```python
from build123d import *

# Parameters (mm, degrees)
F0_W     = 482.6
F0_H     = 88.9
F1_DEPTH = 3
F2_R     = 3
F3_R     = 2.38125
F3_R_2   = 2.246181
F3_R_3   = 2.383077
F3_R_4   = 4.622163
F3_R_5   = 4.540173
F3_R_6   = 3.175
F3_R_7   = 4.7625
F4_DEPTH = 3


with BuildPart() as f1:
    # F0 (on Front) → F1 (new body)
    with BuildSketch(Plane.XZ):
        with Locations((0.070956, -0.013071)):
            Rectangle(F0_W, F0_H)
    extrude(amount=-F1_DEPTH)

    # F2
    f2_edges = [f1.edges().sort_by_distance(p)[0] for p in [
        (-241.229044, 1.5, 44.436929),
        (241.370956, 1.5, 44.436929),
        (241.370956, 1.5, -44.463071),
        (-241.229044, 1.5, -44.463071),
    ]]
    fillet(f2_edges, radius=F2_R)

    # F3 (on Front) → F4 (cut, through all)
    with BuildSketch(Plane.XZ):
        with BuildLine():
            Line((-234.3, 19.186929), (-230.8, 19.186929))
            ThreePointArc((-230.8, 19.186929), (-227.4, 22.586929), (-230.8, 25.986929))
            Line((-230.8, 25.986929), (-234.3, 25.986929))
            ThreePointArc((-234.3, 25.986929), (-237.7, 22.586929), (-234.3, 19.186929))
        make_face()
        with BuildLine():
            ThreePointArc((230.8, 25.986929), (227.4, 22.586929), (230.8, 19.186929))
            Line((230.8, 19.186929), (234.3, 19.186929))
            ThreePointArc((234.3, 19.186929), (237.7, 22.586929), (234.3, 25.986929))
            Line((234.3, 25.986929), (230.8, 25.986929))
        make_face()
        with BuildLine():
            Line((230.8, -25.986929), (234.3, -25.986929))
            ThreePointArc((234.3, -25.986929), (237.7, -22.586929), (234.3, -19.186929))
            Line((234.3, -19.186929), (230.8, -19.186929))
            ThreePointArc((230.8, -19.186929), (227.4, -22.586929), (230.8, -25.986929))
        make_face()
        with BuildLine():
            ThreePointArc((-230.8, -25.986929), (-227.4, -22.586929), (-230.8, -19.186929))
            Line((-230.8, -19.186929), (-234.3, -19.186929))
            ThreePointArc((-234.3, -19.186929), (-237.7, -22.586929), (-234.3, -25.986929))
            Line((-234.3, -25.986929), (-230.8, -25.986929))
        make_face()
        with Locations((-133.35, 13.767754)):
            Circle(F3_R)
        with Locations((-133.35, -5.282246)):
            Circle(F3_R_2)
        with Locations((-133.35, -17.982246)):
            Circle(F3_R_3)
        with Locations((-101.6, -11.684)):
            Circle(F3_R_4)
        with Locations((-82.55, -11.684)):
            Circle(F3_R_5)
        with Locations((-44.45, -11.684)):
            Circle(F3_R_6)
        with Locations((-6.35, -11.684)):
            Circle(F3_R_7)
        with Locations((25.4, -11.684)):
            Circle(F3_R_6)
        with Locations((50.8, -11.684)):
            Circle(F3_R_6)
        with Locations((76.2, -11.684)):
            Circle(F3_R_6)
        with Locations((107.95, -11.684)):
            Circle(F3_R_7)
        with Locations((146.05, -11.684)):
            Circle(F3_R_7)
    extrude(amount=-F4_DEPTH, mode=Mode.SUBTRACT)


solid = f1.part
```
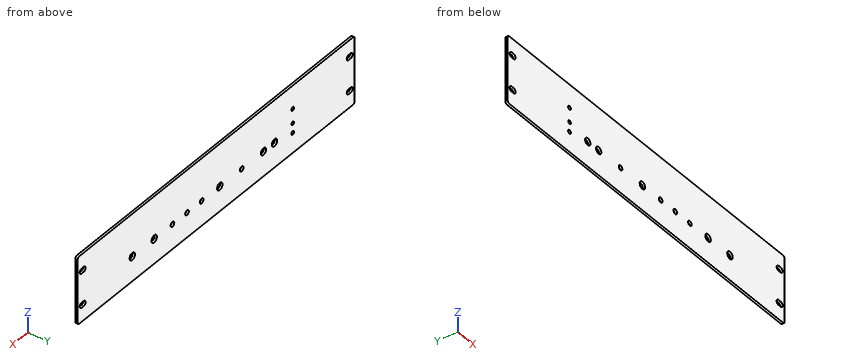
Check sheet for the modelled part. Datum: model origin and axes. Units: mm. Coordinates: 2 decimals unless noted, no trailing zeros. Write each loop counter-clockwise with the first axis right and the second up, starting at its lowest first coordinate (ties: lowest second). Pieces come first, ordered by that corner, then holes. Notation, with made-up numbers: M -22.5,52.25 L 33.5,52.25 A27 cw 33.5,76.25 Z; hole C 39,3 d7. An arc over 180 degrees is marked long. Write item = value, one per line. Start each with the question number.
1. Go/stop test with a flat-tipped pin: pin 1 (3 mm diameter, centred on x = -133.35, z = 13.77, fed in from +Y) (3 decimals). Record where the tip stops, or that it passes through.
2. Sectioned sample at C-C (y = 1). State how many separate pieces and enclosed holes the cut face has, then the cut area to 3 significant figures.
3. Sectioned sample at B-B (x = -6.35). Record the cut outline in (y, z), then the cut area to 3 significant figures.
4. Thickness scan on probe 1 along X at (y, z) = (0.5, -22); probe 2 along Z at (x, y) = (-133.35, 1.2); probe 3 along X at (y, z) = (0.65, -19). Record the ranges inside material, lowest first.
5. Sectioned sample at A-A (x = -82.55). Record the cut outline in (y, z).
The answers:
q1.pin_1 = through
q2.separate_pieces = 1
q2.enclosed_holes = 16
q2.area = 42,100 mm²
q3.outline = M 0,-44.46 L 3,-44.46 L 3,-16.45 L 0,-16.45 Z; M 0,-6.92 L 3,-6.92 L 3,44.44 L 0,44.44 Z
q3.area = 238 mm²
q4.probe_1 = -241.23 to -237.65, -227.45 to 227.45, 237.65 to 241.37
q4.probe_2 = -44.46 to -20.37, -15.6 to -7.53, -3.04 to 11.39, 16.15 to 44.44
q4.probe_3 = -241.23 to -135.5, -131.2 to 241.37
q5.outline = M 0,-44.46 L 3,-44.46 L 3,-16.22 L 0,-16.22 Z; M 0,-7.14 L 3,-7.14 L 3,44.44 L 0,44.44 Z
